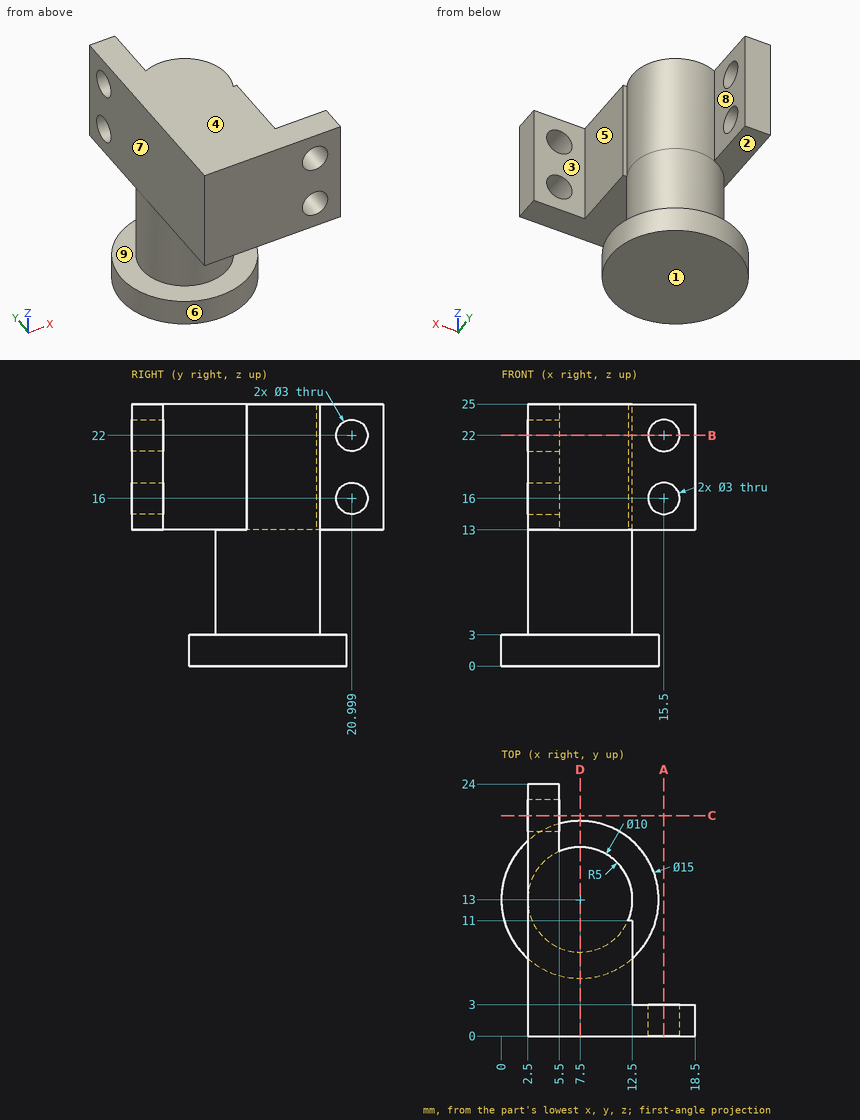
The figure shows three views and two pictorial views of one solid part (mm, origin at its lowest corner). Answer the questions. A direction names the side the tool comes from. Give positions to 0.01 mm unless a question says otherwise; leave off trailing zeros. Write each loop counter-clockwise with the first axis right and the second up, starting at its lowest first coordinate (ties: lowest second). Pieces come first, ordered by that corner, then holes. Notation, with made-up numbers: (34.25, 42) -> (51.25, 42) arc R20 cw to (51.25, 63) -> close; hole circle Ø4 at (82, -34). An arc over 180 degrees is marked (long way). Answer as a JSON object with one key per item and string values.
1) Section D-D on x = 7.5 is taken. Write down the section's boundary in (y, z).
Findings below:
{"outline": "(0, 13) -> (8, 13) -> (8, 3) -> (5.5, 3) -> (5.5, 0) -> (20.5, 0) -> (20.5, 3) -> (18, 3) -> (18, 25) -> (0, 25) -> close"}
2) Straight lines are drawn through the part: probe 1 along Y at (x, z) = (3.75, 22); probe 2 along X at (y, z) = (1.4, 16); probe 3 along Z at (x, y) = (7.5, 7). For each, find the intervals that lie inside material, in ascending order. Write a range as from..to.
Findings below:
{"probe 1": "y = 0..19.5, 22.5..24", "probe 2": "x = 2.5..14, 17..18.5", "probe 3": "z = 0..3, 13..25"}
3) Section B-B on z = 22 is taken. Write down the section's boundary in (x, y).
Findings below:
{"outline": "(2.5, 0) -> (14, 0) -> (14, 3) -> (12.5, 3) -> (12.5, 11) -> (12.08, 11) arc R5 ccw to (5.5, 17.58) -> (5.5, 19.5) -> (2.5, 19.5) -> close; (2.5, 22.5) -> (5.5, 22.5) -> (5.5, 24) -> (2.5, 24) -> close; (17, 0) -> (18.5, 0) -> (18.5, 3) -> (17, 3) -> close"}
4) Flat-ended cylindrical pins translate along their axes: pin 1 Ø3 at (y, z) = (20.5, 18.5) entering from +X; pin 2 Ø13 at (y, z) = (6.5, 21.5) entering from -X; pin 3 Ø0.5 at (x, z) = (12, 17.5) entering from +Y (1 decimal). Find the tip coordinate at first contact, or state that the pin passes through.
Findings below:
{"pin 1": "stops at x = 5.5", "pin 2": "stops at x = 2.5", "pin 3": "stops at y = 15.6"}
5) Section C-C on y = 21 is taken. Write down the section's boundary in (x, z), then the cut area to 3 significant figures.
Findings below:
{"outline": "(2.5, 13) -> (5.5, 13) -> (5.5, 14.5) -> (2.5, 14.5) -> close; (2.5, 17.5) -> (5.5, 17.5) -> (5.5, 20.5) -> (2.5, 20.5) -> close; (2.5, 23.5) -> (5.5, 23.5) -> (5.5, 25) -> (2.5, 25) -> close", "area": "18.0 mm^2"}
6) A tool of negligible diameter and unlimited length cuts with its end or side. For the marked faces 5, 6, 7, 8 and 9, from which of +Z, -Z, +X, -X, +Y, -Y can it reach the whole face along a straight path? Write none if from no direction.
Findings below:
{"face 5": "+Z, +X, +Y", "face 6": "-Z", "face 7": "+Z, -X, +Y, -Y", "face 8": "+Z, +Y", "face 9": "none"}
7) For a pull along Z with two mould halves and no side action, classify the marked faces 1, 2, 3 and 4 as pulls with the +Z half, pulls with the -Z half, needs draft (parallel to the pull), parting line crosses it, or undercut.
Findings below:
{"face 1": "pulls with the -Z half", "face 2": "undercut", "face 3": "needs draft", "face 4": "pulls with the +Z half"}
8) Section A-A on x = 15.5 is taken. Write down the section's boundary in (y, z), then the cut area to 3 significant figures.
Findings below:
{"outline": "(0, 13) -> (3, 13) -> (3, 14.5) -> (0, 14.5) -> close; (0, 17.5) -> (3, 17.5) -> (3, 20.5) -> (0, 20.5) -> close; (0, 23.5) -> (3, 23.5) -> (3, 25) -> (0, 25) -> close", "area": "18.0 mm^2"}
